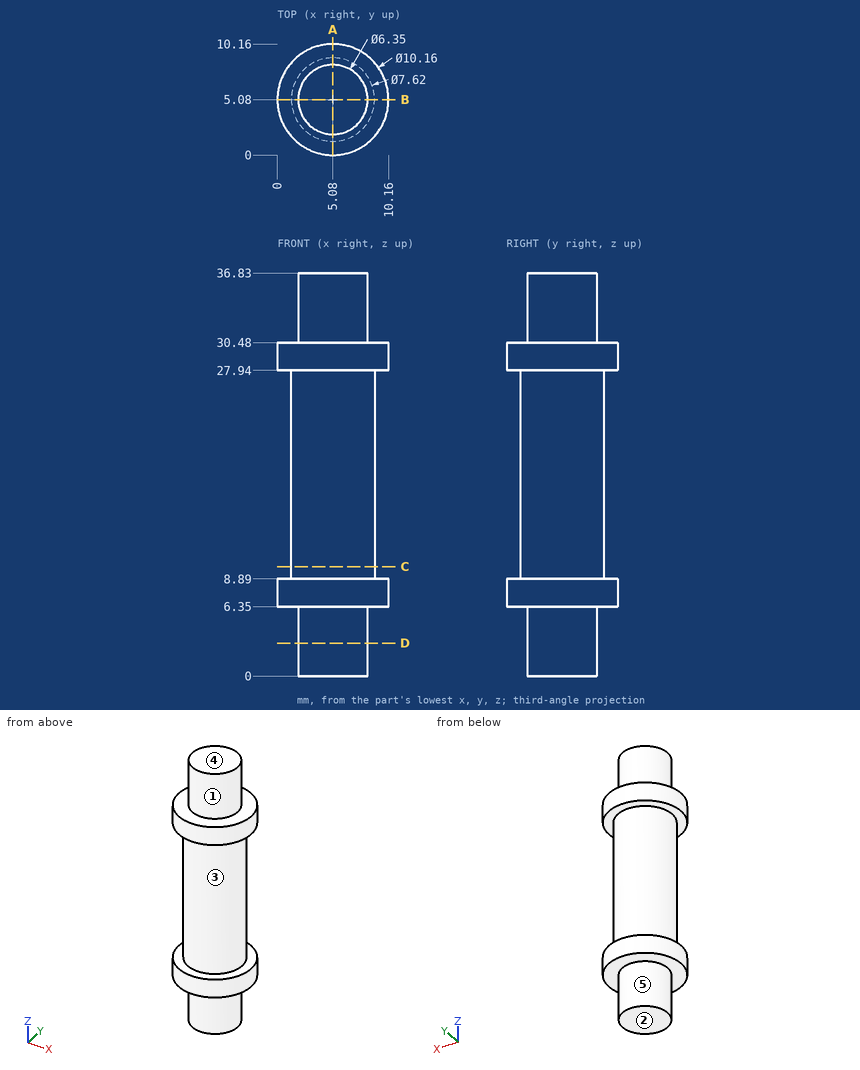
Source: three-view drawing plus pictorial views. Frame: mm from the lowest corner of the part. A direction names the side the tool comes from. Give positions to 0.01 mm unless a question says otherwise; leave off trailing zeros. Order: outer loops, then holes, each group sorted by start corner. A loop starts at its lowest first (then second) coordinate and runs counter-clockwise, first axis right, second up. Notation, with made-up numbers: (18.25, 31.25) -> (70.25, 31.25) arc R8 cw to (70.25, 38.25) -> close; hole circle Ø8 at (-15.5, 53.25). An arc over 180 degrees is marked (long way). Write each question's results on one line, items separated by ' | '. Start each with the question number.
Item 1: Line query: line 1 (Z direction, x = 9, y = 3.75); line 2 (Z direction, x = 3.25, y = 7.75); line 3 (Y direction, x = 3.25, z = 20). Output: solid intervals per line, ascending.
Item 2: Cut plane C-C on z = 10. Return the cut outline in (x, y), then the cut area to 3 significant figures.
Item 3: Set-up query: the marked faces 1, 2, 3, 4 and 5. Return all of +Z, -Z, +X, -X, +Y, -Y with unobstructed straight access to the full face (end or side cutting, diameter ignored); none if empty.
Item 4: Contact query for flat-ended pins moving along their axis: P1, Ø3, axis at x = 7, z = 32.5, coming from the +Y side; P2, Ø1, axis at y = 4, z = 8, coming from the -X side; P3, Ø6, axis at y = 1.5, z = 26.5, coming from the -X side. Output: stop coordinate, or through.
Item 5: Cut plane D-D on z = 3. Return the cut outline in (x, y) (3 decimals).
Item 6: Cut plane A-A on x = 5.08. Return the cut outline in (y, z) (3 decimals), then the cut area to 3 significant figures.
Established:
1) line 1: 6.35 to 8.89, 27.94 to 30.48 | line 2: 6.35 to 30.48 | line 3: 1.74 to 8.42
2) outline: circle Ø7.62 at (5.08, 5.08) | area: 45.6 mm^2
3) face 1: +Z | face 2: -Z, +X, -X, +Y, -Y | face 3: none | face 4: +Z, +X, -X, +Y, -Y | face 5: -Z
4) P1: y = 8.23 | P2: x = 0.03 | P3: x = 0.09
5) outline: circle Ø6.35 at (5.08, 5.08)
6) outline: (0, 6.35) -> (1.905, 6.35) -> (1.905, 0) -> (8.255, 0) -> (8.255, 6.35) -> (10.16, 6.35) -> (10.16, 8.89) -> (8.89, 8.89) -> (8.89, 27.94) -> (10.16, 27.94) -> (10.16, 30.48) -> (8.255, 30.48) -> (8.255, 36.83) -> (1.905, 36.83) -> (1.905, 30.48) -> (0, 30.48) -> (0, 27.94) -> (1.27, 27.94) -> (1.27, 8.89) -> (0, 8.89) -> close | area: 277 mm^2
